```python
from build123d import *

# Parameters (mm, degrees)
SKETCH1_W           = 60
SKETCH1_H           = 60
BOSS_EXTRUDE1_DEPTH = 5
BOSS_EXTRUDE2_DEPTH = 100
SKETCH3_W           = 15
SKETCH3_H           = 15
BOSS_EXTRUDE3_DEPTH = 15
CUT_EXTRUDE1_DEPTH  = 119.11011811
SKETCH5_R           = 3.5
CUT_EXTRUDE2_DEPTH  = 109.627804912
SKETCH6_R           = 5
CUT_EXTRUDE3_DEPTH  = 1
CUT_EXTRUDE4_DEPTH  = 109.627804912


with BuildPart() as part:
    # Sketch1 → Boss-Extrude1 (new body)
    with BuildSketch(Plane(origin=(0, 0, 0), x_dir=(1, 0, 0), z_dir=(0, 1, 0))):
        Rectangle(SKETCH1_W, SKETCH1_H)
    extrude(amount=BOSS_EXTRUDE1_DEPTH)

    # Sketch2 → Boss-Extrude2 (add)
    with BuildSketch(Plane(origin=(0, 5, 0), x_dir=(1, 0, 0), z_dir=(0, 1, 0))):
        Polygon((-30, 30), (-30, 0), (0, 15), (0, 30), align=None)
    extrude(amount=BOSS_EXTRUDE2_DEPTH)

    # Sketch3 → Boss-Extrude3 (add)
    with BuildSketch(Plane(origin=(0, 5, 0), x_dir=(1, 0, 0), z_dir=(0, 1, 0))):
        with Locations((7.5, 22.5)):
            Rectangle(SKETCH3_W, SKETCH3_H)
    extrude(amount=BOSS_EXTRUDE3_DEPTH)

    # Sketch4 → Cut-Extrude1 (cut, through all)
    with BuildSketch(Plane.XY.offset(-15)):
        with BuildLine():
            Line((0, 20), (15, 20))
            Line((15, 20), (15, 5))
            ThreePointArc((15, 5), (4.934047308, 9.934047308), (0, 20))
        make_face()
    extrude(amount=-CUT_EXTRUDE1_DEPTH, mode=Mode.SUBTRACT)

    # Sketch5 → Cut-Extrude2 (cut, through all)
    with BuildSketch(Plane(origin=(0, 5, 0), x_dir=(1, 0, 0), z_dir=(0, 1, 0))):
        with Locations(Location((15, -15, 0), (0, 0, 270))):
            Circle(SKETCH5_R)
    extrude(amount=-CUT_EXTRUDE2_DEPTH, mode=Mode.SUBTRACT)

    # Sketch6 → Cut-Extrude3 (cut)
    with BuildSketch(Plane(origin=(0, 5, 0), x_dir=(1, 0, 0), z_dir=(0, 1, 0))):
        with Locations(Location((15, -15, 0), (0, 0, 270))):
            Circle(SKETCH6_R)
    extrude(amount=-CUT_EXTRUDE3_DEPTH, mode=Mode.SUBTRACT)

    # Sketch7 → Cut-Extrude4 (cut, through all)
    with BuildSketch(Plane(origin=(0, 5, 0), x_dir=(1, 0, 0), z_dir=(0, 1, 0))):
        Polygon((0, 15), (30, 30), (30, 7.119616729), (0, 7.119616729), align=None)
    extrude(amount=CUT_EXTRUDE4_DEPTH, mode=Mode.SUBTRACT)


solid = part.part
```
Part model, mm, in its own coordinate system. A direction names the side the tool comes from. Coordinates: 2 decimals unless noted, no trailing zeros. Write each loop counter-clockwise with the first axis right and the second up, starting at its lowest first coordinate (ties: lowest second). Pieces come first, ordered by that corner, then holes.
Item 1: Slice it at C-C (y = 24.5). Write the cut outline in (x, z), and give its area (3 significant figures).
Item 2: Slice it at D-D (z = -4). Write the cut outline in (x, y).
Item 3: Which spindle directions (+Z, -Z, +X, -X, +Y, -Y) get a long thin tool onto all of the face, cutting with end or side? Do faces 4 (the face through (12.8, 4, 18.3)), 5 (the face through (0, 62, -22)), 6 (the face through (6, 5, 6)). Say none if no direction does.
Item 4: Slice it at B-B (x = -22). Write the cut outline in (y, z), and give its area (3 significant figures).
Item 5: Pin check, flat tips, straight feed: pin 1 (12 mm diameter, centred on y = 62.5, z = 4.5, fed in from +X); pin 2 (5 mm diameter, centred on x = -19, y = 21, fed in from +Z); pin 3 (2 mm diameter, centred on y = 29, z = -19, fed in from +X); pin 4 (5.5 mm diameter, centred on x = 15, z = 15, fed in from -Y). Stop position of each tip, or through.
Item 6: Probe line 1 (X direction, y = 2.4, z = 15); line 2 (X direction, y = 4.8, z = 15); line 3 (Y direction, x = 7.5, z = 14). List the from-to ranges inside material, lowest first.
Item 7: Slice it at A-A (z = 15). Write the cut outline in (x, y), and give its area (3 significant figures).
Item 8: Mould opens along Z. For faces 1 (the face through (-12.8, 54.3, -8.6)), 2 (the face through (10.564, 4.507, 17.307)), 3 (the face through (0, 0, 0)) say: released by +Z, released by -Z, zero draft, split by the parting line, or undercut.
Results found:
1. outline: (-30, -30) - (0, -30) - (0, -15) - (-30, 0) - close
1. area: 675 mm2
2. outline: (-30, 0) - (30, 0) - (30, 5) - (-22, 5) - (-22, 105) - (-30, 105) - close
3. face 4: +Y
3. face 5: +Z, -Z, +X, +Y
3. face 6: +Z, +X, +Y
4. outline: (0, -30) - (105, -30) - (105, -4) - (5, -4) - (5, 30) - (0, 30) - close
4. area: 2,900 mm2
5. pin 1: stops at x = -27
5. pin 2: stops at z = -4.25
5. pin 3: stops at x = 0
5. pin 4: passes through
6. line 1: x = -30 to 11.5, 18.5 to 30
6. line 2: x = -30 to 10, 20 to 30
6. line 3: y = 0 to 5
7. outline: (-30, 0) - (11.5, 0) - (11.5, 4) - (10, 4) - (10, 5) - (-30, 5) - close; (18.5, 0) - (30, 0) - (30, 5) - (20, 5) - (20, 4) - (18.5, 4) - close
7. area: 262 mm2
8. face 1: released by +Z
8. face 2: undercut
8. face 3: zero draft
